Can you work these out from the model? Positions are in its coordinate system, mm. A direction names the side the tool comes from. Give positions to 0.01 mm unless a question says otherwise; leave off trailing zeros. Order: outer loops, then holes, each group sorted by start corner. A loop starts at its lowest first (then second) coordinate and runs counter-clockwise, first axis right, second up. Notation, with made-up numbers: (88.25, 3) -> (98.25, 3) arc R27 ccw to (98.25, 39) -> close; hole circle Ø9 at (-28, -0.75). An arc over 180 degrees is marked (long way). Answer as CSV lines item,"result".
```python
from build123d import *

# Parameters (mm, degrees)
F0_W     = 150
F0_H     = 200
F1_DEPTH = 150
F4_R     = 100
F5_DEPTH = 180


with BuildPart() as f1:
    # F0 (on Top) → F1 (new body)
    with BuildSketch(Plane.XY):
        Rectangle(F0_W, F0_H)
    extrude(amount=F1_DEPTH)

    # F4 (on face) → F5 (cut)
    with BuildSketch(Plane(origin=(0, -89.9519052838, 155.8012701892), x_dir=(1, 0, 0), z_dir=(0, 0.5, -0.8660254038))):
        with Locations((0, -103.3974596216)):
            Circle(F4_R)
    extrude(amount=F5_DEPTH, mode=Mode.SUBTRACT)


solid = f1.part
```
Item 1: Imagine slicing it at A-A, the plane x = -27.5. Please give me the cut outline in (y, z), then the cut area to 3 significant figures.
Numbers:
outline,"(-100, 0) -> (100, 0) -> (100, 57.62) -> (6.33, 3.54) -> (-78.23, 150) -> (-100, 150) -> close"
area,"12,600 mm²"
Item 2: Imagine slicing it at C-C, the plane x = -46. Please give me the cut outline in (y, z).
Numbers:
outline,"(-100, 0) -> (100, 0) -> (100, 57.62) -> (12.7, 7.22) -> (-69.74, 150) -> (-100, 150) -> close"
Item 3: We'd pull the mould along X, two halves only. Please class faces 3 (the flat face through (75, -24, 57)), 4 (the cylindrical face through (1.19, -40.44, 76.85)), 5 (the flat face through (-1, -100, 74)): released by +X, released by -X, zero draft, split by the parting line, or undercut.
Numbers:
face 3,"released by +X"
face 4,"undercut"
face 5,"zero draft"
Item 4: Please list where these lines run through material, in increasing order: line 1 along Y through (x, z) = (-57, 25); line 2 along Y through (x, z) = (-67.5, 39); line 3 along Z through (x, y) = (4, 10).
Numbers:
line 1,"y = -100 to 10.08, 43.49 to 100"
line 2,"y = -100 to 11.68, 67.74 to 100"
line 3,"z = 0 to 5.66"
Item 5: For pin 1 (2 mm diameter, centred on x = 56.5, z = 66, fed in from +Y), with a flat end and sliding along its axis, tell me the tip position at first contact or that it passes through.
Numbers:
pin 1,"stops at y = -13"
Item 6: Imagine slicing it at B-B, the plane y = 47. Please give me the cut outline in (x, z).
Numbers:
outline,"(-75, 0) -> (75, 0) -> (75, 27.02) -> (-75, 27.02) -> close"
Item 7: For faces 1 (the flat face through (-1.05, 50.82, 29.23)), 2 (the flat face through (-1, 100, 28)), which set-ups out of +Z, -Z, +X, -X, +Y, -Y let a thin tool reach every point of the face, with its end or its side?
Numbers:
face 1,"+Z"
face 2,"+Z, -Z, +X, -X, +Y"
